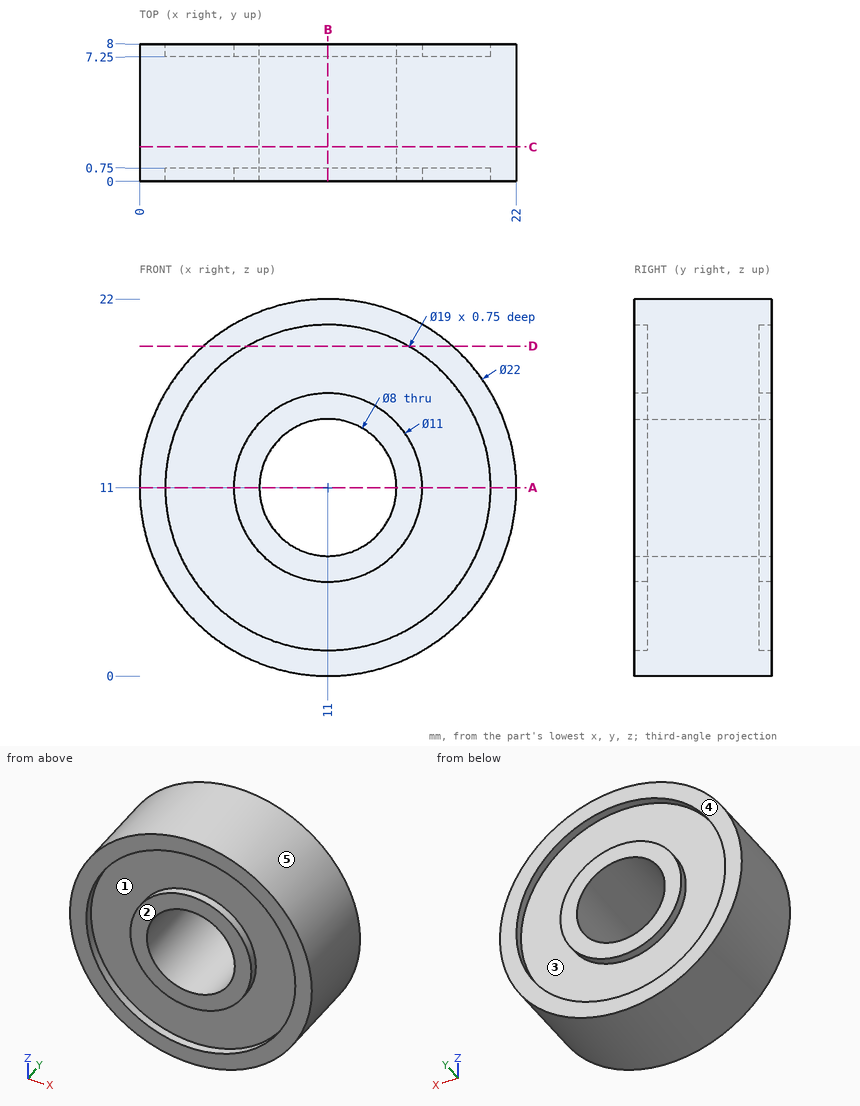
Job drawing, mm, ordinate dimensions from the low corner. One solid piece. A direction names the side the tool comes from. Give positions to 0.01 mm unless a question says otherwise; leave off trailing zeros. Write each loop counter-clockwise with the first axis right and the second up, starting at its lowest first coordinate (ties: lowest second). Pieces come first, ordered by that corner, then holes. Notation, with made-up numbers: (-5, -37.5) -> (23, -37.5) arc R19 cw to (23, -27.5) -> close; hole circle Ø6 at (28.5, -25.5). An arc over 180 degrees is marked (long way). Return JSON: item names as keys, results as strings.
Item 1: Band-saw the part on C-C (y = 2). List the corners of the cut face in (x, z).
Answer below:
{"outline": "circle Ø22 at (11, 11); hole circle Ø8 at (11, 11)"}
Item 2: Two-plate mould, pull along Z, no slides. Class the marked faces 3, 4 and 5: +Z half, -Z half, draft (parallel to the pull), parting line (faces both ways), or undercut.
Answer below:
{"face 3": "undercut", "face 4": "draft", "face 5": "parting line"}
Item 3: Tool access for the marked faces 1 and 2: list every direction of +Z, -Z, +X, -X, +Y, -Y with a clear straight run to the whole face (end or side of a thin tool).
Answer below:
{"face 1": "-Y", "face 2": "+Z, -Z, +X, -X, -Y"}
Item 4: Band-saw the part on B-B (x = 11). List the corners of the cut face in (y, z).
Answer below:
{"outline": "(0, 0) -> (8, 0) -> (8, 1.5) -> (7.25, 1.5) -> (7.25, 5.5) -> (8, 5.5) -> (8, 7) -> (0, 7) -> (0, 5.5) -> (0.75, 5.5) -> (0.75, 1.5) -> (0, 1.5) -> close; (0, 15) -> (8, 15) -> (8, 16.5) -> (7.25, 16.5) -> (7.25, 20.5) -> (8, 20.5) -> (8, 22) -> (0, 22) -> (0, 20.5) -> (0.75, 20.5) -> (0.75, 16.5) -> (0, 16.5) -> close"}
Item 5: Drill centre lines: probe 1 along Z at (x, y) = (11, 0.2); probe 2 along Z at (x, y) = (11, 3); probe 3 along Y at (x, z) = (18.75, 8). Where is each one in solid material? Low to high.
Answer below:
{"probe 1": "z = 0 to 1.5, 5.5 to 7, 15 to 16.5, 20.5 to 22", "probe 2": "z = 0 to 7, 15 to 22", "probe 3": "y = 0.75 to 7.25"}
Item 6: Band-saw the part on D-D (z = 19.25). List the corners of the cut face in (x, y), then the cut area to 3 significant figures.
Answer below:
{"outline": "(3.72, 0) -> (6.29, 0) -> (6.29, 0.75) -> (15.71, 0.75) -> (15.71, 0) -> (18.28, 0) -> (18.28, 8) -> (15.71, 8) -> (15.71, 7.25) -> (6.29, 7.25) -> (6.29, 8) -> (3.72, 8) -> close", "area": "102 mm2"}
Item 7: Drop flat-ended pins along their axis: pin 1 (2 mm diameter, centred on y = 2, z = 15, fed in from -X); pin 2 (2 mm diameter, centred on x = 9, y = 1.5, fed in from +Z); pin 3 (3 mm diameter, centred on x = 14.5, y = 2.5, fed in from +Z). Give the stop position or say it passes through.
Answer below:
{"pin 1": "stops at x = 0.42", "pin 2": "stops at z = 21.95", "pin 3": "stops at z = 21.82"}
Item 8: Band-saw the part on A-A (z = 11). List the corners of the cut face in (x, y).
Answer below:
{"outline": "(0, 0) -> (1.5, 0) -> (1.5, 0.75) -> (5.5, 0.75) -> (5.5, 0) -> (7, 0) -> (7, 8) -> (5.5, 8) -> (5.5, 7.25) -> (1.5, 7.25) -> (1.5, 8) -> (0, 8) -> close; (15, 0) -> (16.5, 0) -> (16.5, 0.75) -> (20.5, 0.75) -> (20.5, 0) -> (22, 0) -> (22, 8) -> (20.5, 8) -> (20.5, 7.25) -> (16.5, 7.25) -> (16.5, 8) -> (15, 8) -> close"}
